Build history of the part. All positions in model axes, mm. Round coordinates to 2 decimals unless told otherwise and drop trailing zeros. Write each loop counter-clockwise with the first axis right and the second up, starting at its lowest first coordinate (ties: lowest second). Pieces come first, ordered by that corner, then holes.
1) Flat gauge pins, fed straight in: pin 1 (5 mm diameter, centred on y = -121.5, z = 3.5, fed in from +X); pin 2 (4.5 mm diameter, centred on x = -157.5, y = -55.64, fed in from -Z); pin 3 (2 mm diameter, centred on x = -230.5, z = 2, fed in from +Y); pin 4 (5 mm diameter, centred on x = -71.5, z = 7.5, fed in from +Y). Where does each tip first touch, or does it go through?
2) Saw through at D-D (x = -250). Write the cut outline in (y, z).
3) Saw through at B-B (z = 6.25). State how many separate pieces and enclosed holes the cut face has, plus the area to 3 significant figures.
4) Saw through at C-C (y = -93.5). Write the cut outline in (x, z).
5) Wall check: probe 1 along Y at (x, z) = (-52.5, 5); probe 2 along Y at (x, z) = (-157.5, 7); probe 3 along Y at (x, z) = (-105, 3). Give the ranges that are in metal, low to high.
6) Saw through at A-A (y = 0). Write the cut outline in (x, z).
from build123d import *

# Parameters (mm, degrees)
ESQUISSE1_R             = 47.5
BOSS_EXTRU_1_DEPTH      = 10
ESQUISSE3_W             = 100
ESQUISSE3_H             = 10
ENL_V_MAT_EXTRU_1_DEPTH = 11
ESQUISSE4_R             = 2.5
ENL_V_MAT_EXTRU_2_DEPTH = 11
ESQUISSE6_W             = 150
ESQUISSE6_H             = 120
BOSS_EXTRU_2_DEPTH      = 10
ESQUISSE7_W             = 10
ESQUISSE7_H             = 50
ESQUISSE7_W_2           = 50
ESQUISSE7_H_2           = 10
ENL_V_MAT_EXTRU_3_DEPTH = 10
ESQUISSE9_W             = 316.248151929
ESQUISSE9_H             = 610.204039151
ENL_V_MAT_EXTRU_4_DEPTH = 10
ESQUISSE10_W            = 334.898216685
ESQUISSE10_H            = 314.009507296
ENL_V_MAT_EXTRU_6_DEPTH = 10
ESQUISSE11_W            = 10
ESQUISSE11_H            = 50
ENL_V_MAT_EXTRU_7_DEPTH = 10


with BuildPart() as part:
    # Esquisse1 → Boss.-Extru.1 (new body)
    with BuildSketch(Plane.XY):
        Polygon((-310, -75.642859016), (0, 414.561180135), (310, -75.642859016), align=None)
        with Locations((-157.5, 0)):
            Circle(ESQUISSE1_R, mode=Mode.SUBTRACT)
        with Locations((-52.5, 0)):
            Circle(ESQUISSE1_R, mode=Mode.SUBTRACT)
        with Locations((52.5, 0)):
            Circle(ESQUISSE1_R, mode=Mode.SUBTRACT)
        with Locations((157.5, 0)):
            Circle(ESQUISSE1_R, mode=Mode.SUBTRACT)
        with Locations((-105, 90.932667397)):
            Circle(ESQUISSE1_R, mode=Mode.SUBTRACT)
        with Locations((0, 90.932667397)):
            Circle(ESQUISSE1_R, mode=Mode.SUBTRACT)
        with Locations((105, 90.932667397)):
            Circle(ESQUISSE1_R, mode=Mode.SUBTRACT)
        with Locations((-52.5, 181.865334795)):
            Circle(ESQUISSE1_R, mode=Mode.SUBTRACT)
        with Locations((52.5, 181.865334795)):
            Circle(ESQUISSE1_R, mode=Mode.SUBTRACT)
        with Locations((0, 272.798002192)):
            Circle(ESQUISSE1_R, mode=Mode.SUBTRACT)
    extrude(amount=BOSS_EXTRU_1_DEPTH)

    # Esquisse3 → Enlèv. mat.-Extru.1 (cut, through all)
    with BuildSketch(Plane.XY.offset(10)):
        Polygon((-269.913793103, -12.254405678), (-261.461999325, -17.599233264), (-208.013723463, 66.918704521), (-216.465517241, 72.263532107), align=None)
        Polygon((-181.724137931, 127.200191667), (-173.272344153, 121.855364081), (-119.82406829, 206.373301865), (-128.275862069, 211.718129452), align=None)
        Polygon((-93.534482759, 266.654789012), (-85.08268898, 261.309961425), (-31.634413118, 345.82789921), (-40.086206897, 351.172726796), align=None)
        Polygon((269.913793103, -12.254405678), (261.461999325, -17.599233264), (208.013723463, 66.918704521), (216.465517241, 72.263532107), align=None)
        Polygon((181.724137931, 127.200191667), (173.272344153, 121.855364081), (119.82406829, 206.373301865), (128.275862069, 211.718129452), align=None)
        Polygon((93.534482759, 266.654789012), (85.08268898, 261.309961425), (31.634413118, 345.82789921), (40.086206897, 351.172726796), align=None)
        with Locations((-160, -70.642859016)):
            Rectangle(ESQUISSE3_W, ESQUISSE3_H)
        with Locations((160, -70.642859016)):
            Rectangle(ESQUISSE3_W, ESQUISSE3_H)
    extrude(amount=-ENL_V_MAT_EXTRU_1_DEPTH, mode=Mode.SUBTRACT)

    # Esquisse4 → Enlèv. mat.-Extru.2 (cut, through all)
    with BuildSketch(Plane.XY.offset(10)):
        with Locations((-157.5, -55.642859016)):
            Circle(ESQUISSE4_R)
        with Locations((-52.5, -55.642859016)):
            Circle(ESQUISSE4_R)
        with Locations((52.5, -55.642859016)):
            Circle(ESQUISSE4_R)
        with Locations((157.5, -55.642859016)):
            Circle(ESQUISSE4_R)
        with Locations((-105, 29.047375097)):
            Circle(ESQUISSE4_R)
        with Locations((0, 29.047375097)):
            Circle(ESQUISSE4_R)
        with Locations((105, 29.047375097)):
            Circle(ESQUISSE4_R)
        with Locations((-52.5, 119.980042494)):
            Circle(ESQUISSE4_R)
        with Locations((52.5, 119.980042494)):
            Circle(ESQUISSE4_R)
        with Locations((0, 210.912709891)):
            Circle(ESQUISSE4_R)
    extrude(amount=-ENL_V_MAT_EXTRU_2_DEPTH, mode=Mode.SUBTRACT)

    # Esquisse6 → Boss.-Extru.2 (add)
    with BuildSketch(Plane.XY.offset(10)):
        with Locations((0, -135.642859016)):
            Rectangle(ESQUISSE6_W, ESQUISSE6_H)
    extrude(amount=-BOSS_EXTRU_2_DEPTH)

    # Esquisse7 → Enlèv. mat.-Extru.3 (cut)
    with BuildSketch(Plane.XY.offset(10)):
        with Locations((-70, -135.642859016)):
            Rectangle(ESQUISSE7_W, ESQUISSE7_H)
        with Locations((0, -190.642859016)):
            Rectangle(ESQUISSE7_W_2, ESQUISSE7_H_2)
        with Locations((70, -135.642859016)):
            Rectangle(ESQUISSE7_W, ESQUISSE7_H)
    extrude(amount=-ENL_V_MAT_EXTRU_3_DEPTH, mode=Mode.SUBTRACT)

    # Esquisse9 → Enlèv. mat.-Extru.4 (cut)
    with BuildSketch(Plane.XY.offset(10)):
        with Locations((158.124075965, 109.45916056)):
            Rectangle(ESQUISSE9_W, ESQUISSE9_H)
    extrude(amount=-ENL_V_MAT_EXTRU_4_DEPTH, mode=Mode.SUBTRACT)

    # Esquisse10 → Enlèv. mat.-Extru.6 (cut)
    with BuildSketch(Plane.XY.offset(10)):
        with Locations((-167.449108343, 266.465933783)):
            Rectangle(ESQUISSE10_W, ESQUISSE10_H)
    extrude(amount=-ENL_V_MAT_EXTRU_6_DEPTH, mode=Mode.SUBTRACT)

    # Esquisse11 → Enlèv. mat.-Extru.7 (cut)
    with BuildSketch(Plane.XY.offset(10)):
        with Locations((-5, -110.642859016)):
            Rectangle(ESQUISSE11_W, ESQUISSE11_H)
    extrude(amount=-ENL_V_MAT_EXTRU_7_DEPTH, mode=Mode.SUBTRACT)


solid = part.part
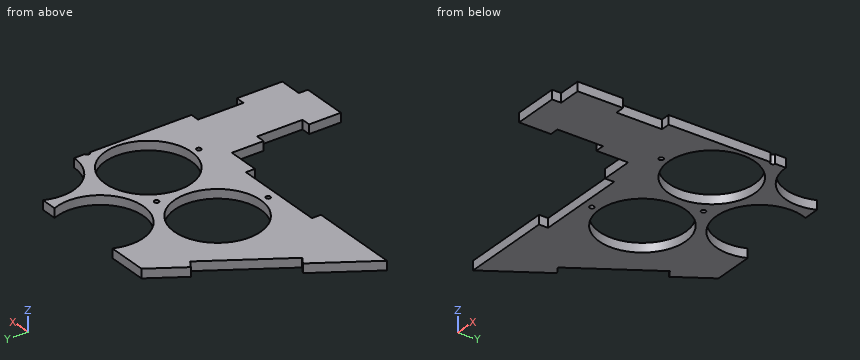
Evaluation:
1. pin 1: stops at x = -10
1. pin 2: passes through
1. pin 3: stops at y = 32.94
1. pin 4: stops at y = 59.94
2. outline: (-75.64, 0) - (0.53, 0) - (0.53, 10) - (-75.64, 10) - close
3. separate pieces: 1
3. enclosed holes: 5
3. area: 30,200 mm2
4. outline: (-75, 0) - (-10, 0) - (-10, 10) - (-75, 10) - close
5. probe 1: y = -195.64 to -58.14, -53.14 to -47.5, 47.5 to 109.46
5. probe 2: y = -65.64 to -58.14, -53.14 to -47.5, 47.5 to 109.46
5. probe 3: y = -75.64 to 26.55, 31.55 to 43.43
6. outline: (-250.33, 0) - (-205, 0) - (-205, 10) - (-250.33, 10) - close; (-110, 0) - (-100, 0) - (-100, 10) - (-110, 10) - close; (-5, 0) - (0, 0) - (0, 10) - (-5, 10) - close
